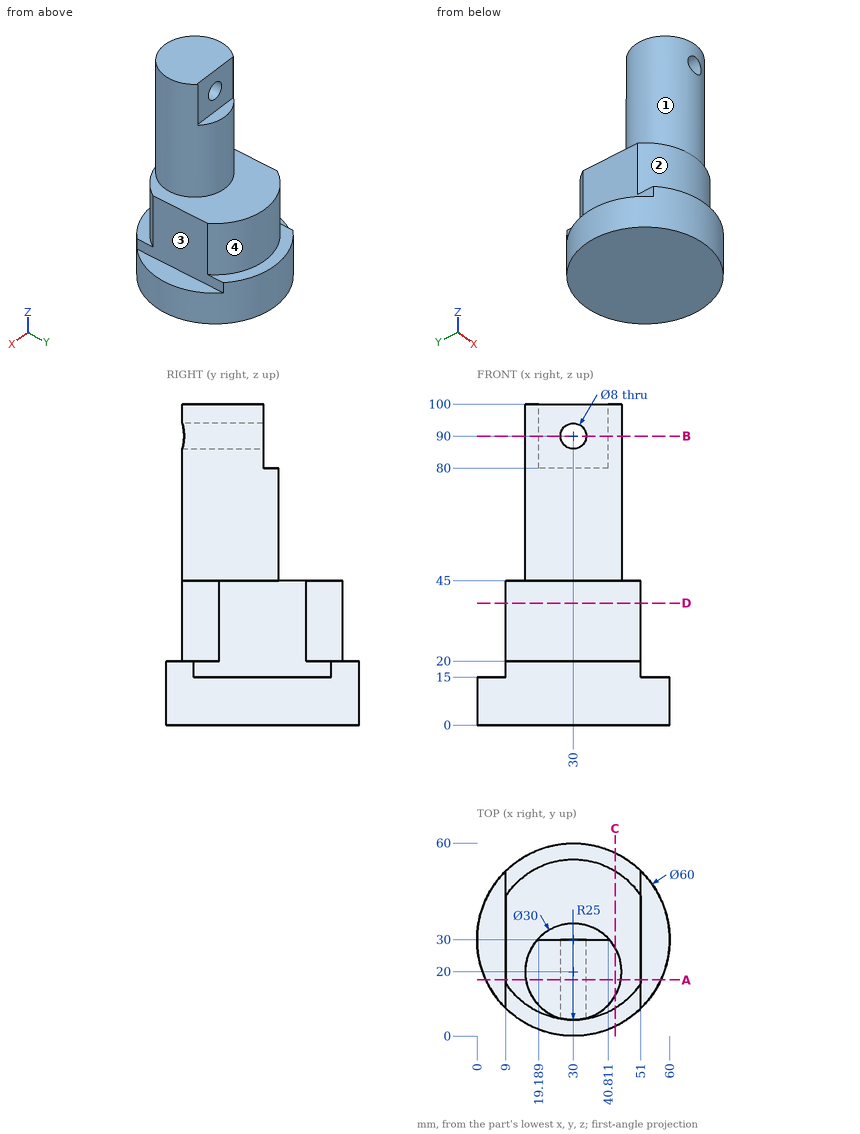
Geometry: see drawing. Coordinates: mm, zero at the bounding-box minimum. A direction names the side the tool comes from. Give positions to 0.01 mm unless a question says otherwise; leave off trailing zeros. Loops run counter-clockwise (first coordinate to the right, second up) from the corner with the lowest first, then second, coordinate; pieces in that order, holes last. Notation, with made-up numbers: (-24.5, 76) - (-11.5, 76) arc R33 ccw to (-11.5, 111) - close; hole circle Ø11 at (44.5, -39). An arc over 180 degrees is marked (long way). Use CSV: the item, a comma, the result in double quotes. Start each with the question number.
Item 1: Section C-C on x = 43. Return loops of the section in (y, z).
Item 2: Section B-B on z = 90. Return loops of the section in (x, y), then the cut area to 3 significant figures.
Item 3: Section D-D on z = 38. Return loops of the section in (x, y) (1 decimal).
Item 4: Section A-A on y = 17.5. Return loops of the section in (x, z), then the cut area to 4 significant figures.
Item 5: Contact query for flat-ended pins moving along their axis: P1, Ø10, axis at y = 22.5, z = 32.5, coming from the +X side; P2, Ø5, axis at x = 22.5, z = 68, coming from the -Y side; P3, Ø9, axis at x = 30, z = 90, coming from the +Y side. Output: stop coordinate, or through.
Item 6: Reachability of the marked faces 1, 2, 3 and 4 from +Z, -Z, +X, -X, +Y, -Y: full face, straight path, thin tool, end or side. Return the list, or none.
Item 7: Line query: line 1 (Z direction, x = 30, y = 22); line 2 (X direction, y = 19.75, z = 90); line 3 (Z direction, x = 44.5, y = 30.5). Output: solid intervals per line, ascending.
Ans:
1,outline,"(2.96, 0) - (57.04, 0) - (57.04, 20) - (51.35, 20) - (51.35, 45) - (27.48, 45) - (27.48, 100) - (12.52, 100) - (12.52, 45) - (8.65, 45) - (8.65, 20) - (2.96, 20) - close"
2,outline,"(19.19, 30) - (19.19, 30.4) arc R15 ccw to (26, 5.54) - (26, 30) - close; (34, 5.54) arc R15 ccw to (40.81, 30.4) - (40.81, 30) - (34, 30) - close"
2,area,"431 mm2"
3,outline,"(9, 16.4) arc R25 ccw to (51, 16.4) - (51, 43.6) arc R25 ccw to (9, 43.6) - close"
4,outline,"(2.73, 0) - (57.27, 0) - (57.27, 15) - (51, 15) - (51, 45) - (44.79, 45) - (44.79, 100) - (15.21, 100) - (15.21, 45) - (9, 45) - (9, 15) - (2.73, 15) - close; hole circle Ø8 at (30, 90)"
4,area,"3,655 mm2"
5,P1,"stops at x = 51"
5,P2,"stops at y = 5.86"
5,P3,"stops at y = 30"
6,face 1,"+Z"
6,face 2,"+Z, -Y"
6,face 3,"+Z, +X, +Y, -Y"
6,face 4,"+Z, +Y"
7,line 1,"z = 0 to 86, 94 to 100"
7,line 2,"x = 15 to 26, 34 to 45"
7,line 3,"z = 0 to 45"
